Design review of the part built by this model. Coordinates are the model's own, in mm. Coordinates: 2 decimals unless noted, no trailing zeros. Write each loop counter-clockwise with the first axis right and the second up, starting at its lowest first coordinate (ties: lowest second). Pieces come first, ordered by that corner, then holes. Notation, with made-up numbers: (28, 86) - (47, 86) arc R9 cw to (47, 93) - close; hole circle Ø1 at (82.25, 74). An arc over 180 degrees is marked (long way). One line per item, written item: value.
from build123d import *

# Parameters (mm, degrees)
SKETCH1_W           = 139.7
SKETCH1_H           = 101.6
BOSS_EXTRUDE1_DEPTH = 4.7625
SKETCH2_W           = 4.7625
SKETCH2_H           = 101.6
CUT_EXTRUDE1_DEPTH  = 87.500542809
LPATTERN1_COUNT     = 3
LPATTERN1_PITCH     = 57.15


with BuildPart() as part:
    # Sketch1 → Boss-Extrude1 (new body)
    with BuildSketch(Plane.XY):
        Rectangle(SKETCH1_W, SKETCH1_H)
    extrude(amount=BOSS_EXTRUDE1_DEPTH)

    # Sketch2 → Cut-Extrude1 (cut, through all)
    with BuildSketch(Plane.XY.offset(4.7625)):
        with Locations((-57.15, -50.8)):
            Rectangle(SKETCH2_W, SKETCH2_H)
    cut_extrude1 = extrude(amount=-CUT_EXTRUDE1_DEPTH, mode=Mode.SUBTRACT)

    # LPattern1: Cut-Extrude1 ×3
    with Locations(*[(i * LPATTERN1_PITCH, 0, 0) for i in range(1, LPATTERN1_COUNT)]):
        add(cut_extrude1, mode=Mode.SUBTRACT)


solid = part.part
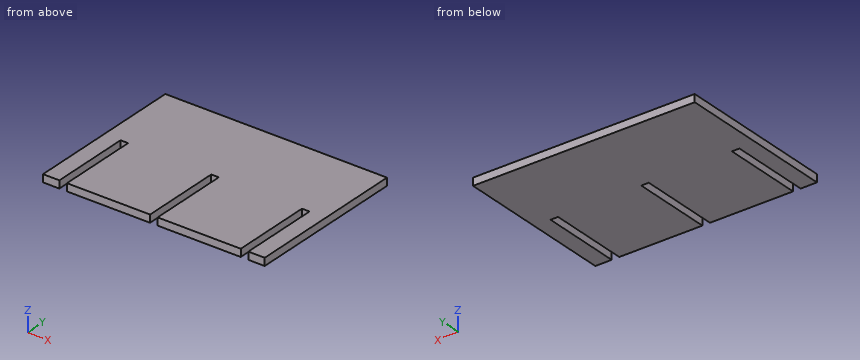
1. Insertion check: pin 1 Ø1.4 at (x, z) = (56, 1) entering from -Y. The pin has a flat end and moves straight along its axis. Give the tip position at first contact, or say it passes through.
Answer block:
pin 1: stops at y = 0
2. Consider section B-B, the plane z = 2.45. Write out the cut boundary in (x, y), then the cut area to 3 significant figures.
Answer block:
outline: (-69.85, -50.8) - (-59.53, -50.8) - (-59.53, 0) - (-54.77, 0) - (-54.77, -50.8) - (-2.38, -50.8) - (-2.38, 0) - (2.38, 0) - (2.38, -50.8) - (54.77, -50.8) - (54.77, 0) - (59.53, 0) - (59.53, -50.8) - (69.85, -50.8) - (69.85, 50.8) - (-69.85, 50.8) - close
area: 13,500 mm^2
3. Wall thickness on line 1 along X through (y, z) = (-40, 1.5); line 2 along Y through (x, z) = (-56, 2.95): over which ranges is each line inside the solid? List them lowest first.
Answer block:
line 1: x = -69.85 to -59.53, -54.77 to -2.38, 2.38 to 54.77, 59.53 to 69.85
line 2: y = 0 to 50.8
4. Consider section A-A, the plane y = -25.5. Write out the cut boundary in (x, z), then the cut area to 3 significant figures.
Answer block:
outline: (-69.85, 0) - (-59.53, 0) - (-59.53, 4.76) - (-69.85, 4.76) - close; (-54.77, 0) - (-2.38, 0) - (-2.38, 4.76) - (-54.77, 4.76) - close; (2.38, 0) - (54.77, 0) - (54.77, 4.76) - (2.38, 4.76) - close; (59.53, 0) - (69.85, 0) - (69.85, 4.76) - (59.53, 4.76) - close
area: 597 mm^2
